```python
from build123d import *

# Parameters (mm, degrees)
BOSS_EXTRUDE1_DEPTH = 12
SKETCH3_R           = 3.6
CUT_EXTRUDE1_DEPTH  = 31.934770082
SKETCH5_R           = 1.75
CUT_EXTRUDE2_DEPTH  = 30.732137495
FILLET1_R           = 1


with BuildPart() as part:
    # Sketch2 → Boss-Extrude1 (new body)
    with BuildSketch(Plane.XY):
        Polygon((-5, 0), (5, 0), (5, -22), (16, -22), (16, -20.4), (6.2, -20.4), (6.2, 1.6), (-6.2, 1.6), (-6.2, -20.4), (-16, -20.4), (-16, -22), (-5, -22), align=None)
    extrude(amount=BOSS_EXTRUDE1_DEPTH)

    # Sketch3 → Cut-Extrude1 (cut, through all)
    with BuildSketch(Plane(origin=(0, 1.6, 0), x_dir=(1, 0, 0), z_dir=(0, 1, 0))):
        with Locations(Location((0, -6, 0), (0, 0, 180))):
            Circle(SKETCH3_R)
    extrude(amount=-CUT_EXTRUDE1_DEPTH, mode=Mode.SUBTRACT)

    # Sketch5 → Cut-Extrude2 (cut, through all)
    with BuildSketch(Plane(origin=(0, -20.4, 0), x_dir=(1, 0, 0), z_dir=(0, 1, 0))):
        with Locations(Location((-10, -6, 0), (0, 0, 180))):
            Circle(SKETCH5_R)
        with Locations(Location((10, -6, 0), (0, 0, 180))):
            Circle(SKETCH5_R)
    extrude(amount=-CUT_EXTRUDE2_DEPTH, mode=Mode.SUBTRACT)

    # Fillet1
    # the kernel refuses this fillet: 1 mm, written as the material it adds along each edge
    with BuildSketch(Plane(origin=(-6.2, -20.4, 0), x_dir=(0, 1, 0), z_dir=(0, 0, 1)), Plane(origin=(6.2, -20.4, 0), x_dir=(1, 0, 0), z_dir=(0, 0, 1))) as fillet1_piece_1:
        with BuildLine():
            CenterArc((FILLET1_R, FILLET1_R), FILLET1_R, 180, 90)
            Line((0, FILLET1_R), (0, 0))
            Line((0, 0), (FILLET1_R, 0))
        make_face()
    extrude(amount=12)
    # the kernel refuses this fillet: 1 mm, written as the material it takes off along each edge
    with BuildSketch(Plane(origin=(16, -20.4, -2.5), x_dir=(0, -1, 0), z_dir=(0, 0, 1)), Plane(origin=(16, -22, -2.5), x_dir=(-1, 0, 0), z_dir=(0, 0, 1)), Plane(origin=(-16, -20.4, -2.5), x_dir=(1, 0, 0), z_dir=(0, 0, 1)), Plane(origin=(-6.2, 1.6, -2.5), x_dir=(1, 0, 0), z_dir=(0, 0, 1)), Plane(origin=(6.2, 1.6, -2.5), x_dir=(0, -1, 0), z_dir=(0, 0, 1)), Plane(origin=(5, -22, -2.5), x_dir=(0, 1, 0), z_dir=(0, 0, 1))) as fillet1_2_piece_1:
        with BuildLine():
            CenterArc((FILLET1_R, -FILLET1_R), FILLET1_R, 90, 90)
            Line((0, -FILLET1_R), (0, 0))
            Line((0, 0), (FILLET1_R, 0))
        make_face()
    extrude(amount=17, mode=Mode.SUBTRACT)
    with BuildSketch(Plane(origin=(-16, -22, -2.5), x_dir=(1, 0, 0), z_dir=(0, 0, 1)), Plane(origin=(-5, -22, -2.5), x_dir=(0, 1, 0), z_dir=(0, 0, 1))) as fillet1_2_piece_2:
        with BuildLine():
            CenterArc((FILLET1_R, FILLET1_R), FILLET1_R, 180, 90)
            Line((0, FILLET1_R), (0, 0))
            Line((0, 0), (FILLET1_R, 0))
        make_face()
    extrude(amount=17, mode=Mode.SUBTRACT)


solid = part.part
```
Here's how the part is built. I have some questions about the finished solid (model axes, mm). A direction names the side the tool comes from. Coordinates: 2 decimals unless noted, no trailing zeros. Write each loop counter-clockwise with the first axis right and the second up, starting at its lowest first coordinate (ties: lowest second). Pieces come first, ordered by that corner, then holes. Notation, with made-up numbers: (87, 28) - (99, 28) arc R19 cw to (99, 56) - close; hole circle Ø10 at (-11.75, 59). An arc over 180 degrees is marked (long way). One line per item, written item: value.
1) We'd pull the mould along X, two halves only. Please class faces 1 (the cylindrical face through (5.285, -21.699, 5.916)), 2 (the cylindrical face through (5.915, 1.299, 5.916)), 3 (the flat face through (-6, -12, 12)): pulls with the +X half, pulls with the -X half, needs draft (parallel to the pull), parting line crosses it, or undercut.
Model answer:
face 1: undercut
face 2: pulls with the +X half
face 3: needs draft
2) Suppose I cut it at B-B on z = 6. State how many separate pieces and enclosed holes the cut face has, and give its area (3 significant figures).
Model answer:
separate pieces: 4
enclosed holes: 0
area: 80.0 mm²
3) Suppose I cut it at C-C on y = -16. Write out the boundary of the cut face in (x, z).
Model answer:
outline: (-6.2, 0) - (-5, 0) - (-5, 12) - (-6.2, 12) - close; (5, 0) - (6.2, 0) - (6.2, 12) - (5, 12) - close
4) I'm going to push flat-ended pins straight in: P1, Ø6, axis at x = -11, z = 4.5, coming from the +Y side; P2, Ø1, axis at y = -1.5, z = 3.5, coming from the +X side; P3, Ø1.5, axis at x = 10, z = 6, coming from the +Y side; P4, Ø3, axis at y = -14.5, z = 3, coming from the -X side. Where does each tip first touch, or does it pass through?
Model answer:
P1: stops at y = -20.4
P2: stops at x = 6.2
P3: passes through
P4: stops at x = -6.2
5) On a 3-axis mill with a long thin cutter (end or side, diameter ignored), from which of +Z, -Z, +X, -X, +Y, -Y can I reach the whole of each face in a straight line? I mean faces 4 (the flat face through (-12, -20.4, 6)), 5 (the flat face through (12, -20.4, 6)), 6 (the flat face through (11.4, -22, 4.6)), 7 (the flat face through (4, 1.6, 5)), 8 (the flat face through (5, -10, 6)). Say none if no direction works.
Model answer:
face 4: +Z, -Z, -X, +Y
face 5: +Z, -Z, +X, +Y
face 6: +Z, -Z, +X, -X, -Y
face 7: +Z, -Z, +X, -X, +Y
face 8: +Z, -Z, -Y
6) Suppose I cut it at D-D on z = 1.5. Write out the boundary of the cut face in (x, y).
Model answer:
outline: (-15.98, -21.2) arc R1 ccw to (-15, -22) - (-6, -22) arc R1 ccw to (-5, -21) - (-5, 0) - (5, 0) - (5, -21) arc R1 ccw to (6, -22) - (15, -22) arc R1 ccw to (15.98, -21.2) arc R1 ccw to (15, -20.4) - (7.2, -20.4) arc R1 cw to (6.2, -19.4) - (6.2, 0.6) arc R1 ccw to (5.2, 1.6) - (-5.2, 1.6) arc R1 ccw to (-6.2, 0.6) - (-6.2, -19.4) arc R1 cw to (-7.2, -20.4) - (-15, -20.4) arc R1 ccw to start
7) I need wall thicknesses on line 1 along X through (y, z) = (-9, 4); line 2 along Z through (x, y) = (-10, -21.6); line 3 along Y through (x, z) = (13, 3.25). Which ranges of each line are inside material? Lowest first, please.
Model answer:
line 1: x = -6.2 to -5, 5 to 6.2
line 2: z = 0 to 4.25, 7.75 to 12
line 3: y = -22 to -20.4
8) Suppose I cut it at A-A on x = 0. Write out the boundary of the cut face in (y, z), and give its area (3 significant figures).
Model answer:
outline: (0, 0) - (1.6, 0) - (1.6, 2.4) - (0, 2.4) - close; (0, 9.6) - (1.6, 9.6) - (1.6, 12) - (0, 12) - close
area: 7.68 mm²
